Check sheet for the modelled part. Datum: model origin and axes. Units: mm. Round coordinates to 2 decimals unless told otherwise and drop trailing zeros. Write each loop counter-clockwise with the first axis right and the second up, starting at its lowest first coordinate (ties: lowest second). Pieces come first, ordered by that corner, then holes. Notation, with made-up numbers: (-17.75, -3.5) -> (21.25, -3.5) arc R23 cw to (21.25, 32.5) -> close; hole circle Ø1 at (58, 22). An arc over 180 degrees is marked (long way). Write item = value, one per line.
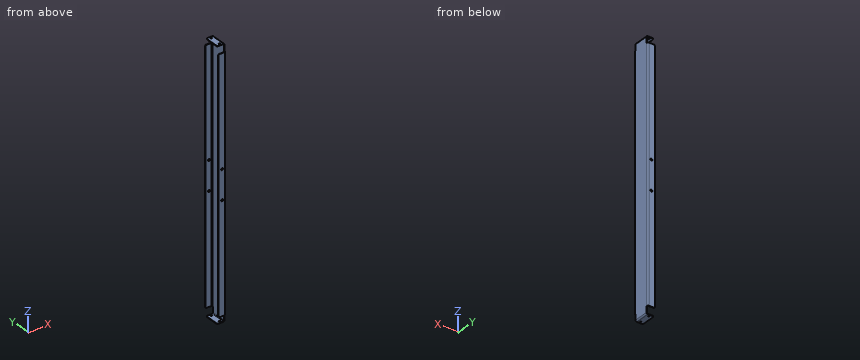
from build123d import *

# Parameters (mm, degrees)
SKETCH1_W                      = 861.06
SKETCH1_H                      = 63.5
BASE_FLANGE1_DEPTH             = 1.89738
EDGE_FLANGE1_STRIP_W           = 12.66952
EDGE_FLANGE1_STRIP_H           = 1.89738
EDGE_FLANGE1_STRIP_CUT_DEPTH   = 861.06
EDGE_FLANGE1_STRIP_2_W         = 12.66952
EDGE_FLANGE1_STRIP_2_H         = 1.89738
EDGE_FLANGE1_STRIP_CUT_2_DEPTH = 861.06
EDGE_FLANGE1_DEPTH             = 861.06
EDGE_FLANGE1_BEND_DEPTH        = 861.06
SKETCH12_W                     = 24.765
SKETCH12_H                     = 50.8
BOSS_EXTRUDE1_DEPTH            = 1.89738
SKETCH13_R                     = 3.3655
CUT_EXTRUDE1_DEPTH             = 461.403026733
EDGE_FLANGE2_STRIP_W           = 12.66952
EDGE_FLANGE2_STRIP_H           = 1.89738
EDGE_FLANGE2_STRIP_CUT_DEPTH   = 50.8
EDGE_FLANGE2_STRIP_2_W         = 12.66952
EDGE_FLANGE2_STRIP_2_H         = 1.89738
EDGE_FLANGE2_STRIP_CUT_2_DEPTH = 50.8
EDGE_FLANGE2_DEPTH             = 50.8
EDGE_FLANGE2_BEND_DEPTH        = 50.8
SKETCH20_R                     = 2.4638
CUT_EXTRUDE2_DEPTH             = 914.154728455
CHAMFER1_SIZE                  = 2.54


# Sheet-metal steps are written as plain solids
with BuildPart() as part:
    # Sketch1 → Base-Flange1 (new body)
    with BuildSketch(Plane(origin=(0, 0, 0), x_dir=(0, 0, -1), z_dir=(1, 0, 0))):
        with Locations((0, 31.75)):
            Rectangle(SKETCH1_W, SKETCH1_H)
    extrude(amount=-BASE_FLANGE1_DEPTH)

    # Edge-Flange1 strip (across the edge) → Edge-Flange1 strip cut (cut)
    with BuildSketch(Plane(origin=(-1.89738, 63.5, 430.53), x_dir=(0, -1, 0), z_dir=(0, 0, -1))):
        with Locations((-1.89738, -0.94869)):
            Rectangle(EDGE_FLANGE1_STRIP_W, EDGE_FLANGE1_STRIP_H)
    extrude(amount=EDGE_FLANGE1_STRIP_CUT_DEPTH, mode=Mode.SUBTRACT)

    # Edge-Flange1 strip 2 (across the edge) → Edge-Flange1 strip cut 2 (cut)
    with BuildSketch(Plane(origin=(-1.89738, 0, -430.53), x_dir=(0, 1, 0), z_dir=(0, 0, 1))):
        with Locations((-1.89738, -0.94869)):
            Rectangle(EDGE_FLANGE1_STRIP_2_W, EDGE_FLANGE1_STRIP_2_H)
    extrude(amount=EDGE_FLANGE1_STRIP_CUT_2_DEPTH, mode=Mode.SUBTRACT)

    # Edge-Flange1 section (across the edge) → Edge-Flange1 (add)
    with BuildSketch(Plane(origin=(-1.89738, 63.5, 430.53), x_dir=(0, -1, 0), z_dir=(0, 0, -1))):
        with BuildLine():
            Line((0, 2.54), (0, 23.50262))
            Line((0, 23.50262), (1.89738, 23.50262))
            Line((1.89738, 23.50262), (1.89738, 2.54))
            ThreePointArc((1.89738, 2.54), (2.641328776, 0.743948776), (4.43738, 0))
            Line((4.43738, 0), (4.43738, -1.89738))
            ThreePointArc((4.43738, -1.89738), (1.299678511, -0.597701489), (0, 2.54))
        make_face()
    extrude(amount=EDGE_FLANGE1_DEPTH)

    # Edge-Flange1 section 2 (across the edge) → Edge-Flange1 bend (add)
    with BuildSketch(Plane(origin=(-1.89738, 0, -430.53), x_dir=(0, 1, 0), z_dir=(0, 0, 1))):
        with BuildLine():
            Line((0, 2.54), (0, 23.50262))
            Line((0, 23.50262), (1.89738, 23.50262))
            Line((1.89738, 23.50262), (1.89738, 2.54))
            ThreePointArc((1.89738, 2.54), (2.641328776, 0.743948776), (4.43738, 0))
            Line((4.43738, 0), (4.43738, -1.89738))
            ThreePointArc((4.43738, -1.89738), (1.299678511, -0.597701489), (0, 2.54))
        make_face()
    extrude(amount=EDGE_FLANGE1_BEND_DEPTH)

    # Sketch12 → Boss-Extrude1 (add)
    with BuildSketch(Plane(origin=(0, 0, 0), x_dir=(0, 0, -1), z_dir=(1, 0, 0))):
        with Locations((-442.9125, 31.75)):
            Rectangle(SKETCH12_W, SKETCH12_H)
    boss_extrude1 = extrude(amount=-BOSS_EXTRUDE1_DEPTH)

    # Mirror1: Boss-Extrude1 across plane
    add(boss_extrude1.mirror(Plane.XY))

    # Sketch13 → Cut-Extrude1 (cut, through all)
    with BuildSketch(Plane(origin=(0, 63.5, 0), x_dir=(1, 0, 0), z_dir=(0, 1, 0))):
        with Locations(Location((-12.7, 50.8, 0), (0, 0, 180))):
            Circle(SKETCH13_R)
        with Locations(Location((-12.7, -50.8, 0), (0, 0, 180))):
            Circle(SKETCH13_R)
    extrude(amount=-CUT_EXTRUDE1_DEPTH, mode=Mode.SUBTRACT)

    # Edge-Flange2 strip (across the edge) → Edge-Flange2 strip cut (cut)
    with BuildSketch(Plane(origin=(-1.89738, 6.35, 455.295), x_dir=(0, 0, -1), z_dir=(0, 1, 0))):
        with Locations((-1.89738, -0.94869)):
            Rectangle(EDGE_FLANGE2_STRIP_W, EDGE_FLANGE2_STRIP_H)
    extrude(amount=EDGE_FLANGE2_STRIP_CUT_DEPTH, mode=Mode.SUBTRACT)

    # Edge-Flange2 strip 2 (across the edge) → Edge-Flange2 strip cut 2 (cut)
    with BuildSketch(Plane(origin=(-1.89738, 57.15, -455.295), x_dir=(0, 0, 1), z_dir=(0, -1, 0))):
        with Locations((-1.89738, -0.94869)):
            Rectangle(EDGE_FLANGE2_STRIP_2_W, EDGE_FLANGE2_STRIP_2_H)
    extrude(amount=EDGE_FLANGE2_STRIP_CUT_2_DEPTH, mode=Mode.SUBTRACT)

    # Edge-Flange2 section (across the edge) → Edge-Flange2 (add)
    with BuildSketch(Plane(origin=(-1.89738, 6.35, 455.295), x_dir=(0, 0, -1), z_dir=(0, 1, 0))):
        with BuildLine():
            Line((0, 2.54), (0, 23.50262))
            Line((0, 23.50262), (1.89738, 23.50262))
            Line((1.89738, 23.50262), (1.89738, 2.54))
            ThreePointArc((1.89738, 2.54), (2.641328776, 0.743948776), (4.43738, 0))
            Line((4.43738, 0), (4.43738, -1.89738))
            ThreePointArc((4.43738, -1.89738), (1.299678511, -0.597701489), (0, 2.54))
        make_face()
    extrude(amount=EDGE_FLANGE2_DEPTH)

    # Edge-Flange2 section 2 (across the edge) → Edge-Flange2 bend (add)
    with BuildSketch(Plane(origin=(-1.89738, 57.15, -455.295), x_dir=(0, 0, 1), z_dir=(0, -1, 0))):
        with BuildLine():
            Line((0, 2.54), (0, 23.50262))
            Line((0, 23.50262), (1.89738, 23.50262))
            Line((1.89738, 23.50262), (1.89738, 2.54))
            ThreePointArc((1.89738, 2.54), (2.641328776, 0.743948776), (4.43738, 0))
            Line((4.43738, 0), (4.43738, -1.89738))
            ThreePointArc((4.43738, -1.89738), (1.299678511, -0.597701489), (0, 2.54))
        make_face()
    extrude(amount=EDGE_FLANGE2_BEND_DEPTH)

    # Sketch20 → Cut-Extrude2 (cut, through all)
    with BuildSketch(Plane.XY.offset(455.295)):
        with Locations((-12.7, 50.8)):
            Circle(SKETCH20_R)
        with Locations((-12.7, 12.7)):
            Circle(SKETCH20_R)
    extrude(amount=-CUT_EXTRUDE2_DEPTH, mode=Mode.SUBTRACT)

    # Chamfer1
    chamfer1_edges = [part.edges().sort_by_distance(p)[0] for p in [
        (-25.4, 6.35, 454.34631),
        (-25.4, 57.15, 454.34631),
        (-25.4, 57.15, -454.34631),
        (-25.4, 6.35, -454.34631),
        (-25.4, 62.55131, 430.53),
        (-25.4, 62.55131, -430.53),
        (-25.4, 0.94869, -430.53),
        (-25.4, 0.94869, 430.53),
    ]]
    chamfer(chamfer1_edges, length=CHAMFER1_SIZE)


solid = part.part
(1) Material ranges on L1, parallel to Y at x = -12.7, z = 454.7; L2, parallel to Z at x = -12.7, y = 0.95; L3, parallel to Y at x = -7.5, z = -47, recorded low to high. Write a range as [from, to].
Worked answers:
L1 = [6.35, 10.24], [15.16, 48.34], [53.26, 57.15]
L2 = [-430.53, -54.17], [-47.43, 47.43], [54.17, 430.53]
L3 = [0, 1.9], [61.6, 63.5]
(2) Sectioned sample at B-B on y = 32. Enter the section's corners in (x, z) (3 decimals), then the cut area to 3 significant figures.
Worked answers:
outline = (-25.4, -455.295) -> (-4.437, -455.295) arc R4.437 ccw to (0, -450.858) -> (0, 450.858) arc R4.437 ccw to (-4.437, 455.295) -> (-25.4, 455.295) -> (-25.4, 453.398) -> (-4.437, 453.398) arc R2.54 cw to (-1.897, 450.858) -> (-1.897, -450.858) arc R2.54 cw to (-4.437, -453.398) -> (-25.4, -453.398) -> close
area = 1,810 mm²
(3) Go/stop test with flat-tipped pins: P1, Ø4.5, axis at x = -12.7, y = 50.8, coming from the +Z side; P2, Ø3, axis at y = 33.5, z = 101, coming from the -X side. Record where each tip stops, or that it passes through.
Worked answers:
P1 = through
P2 = -1.9
(4) Sectioned sample at A-A on z = -79. Enter the section's corners in (x, y), then the cut area to 3 significant figures.
Worked answers:
outline = (-25.4, 0) -> (-4.44, 0) arc R4.44 ccw to (0, 4.44) -> (0, 59.06) arc R4.44 ccw to (-4.44, 63.5) -> (-25.4, 63.5) -> (-25.4, 61.6) -> (-4.44, 61.6) arc R2.54 cw to (-1.9, 59.06) -> (-1.9, 4.44) arc R2.54 cw to (-4.44, 1.9) -> (-25.4, 1.9) -> close
area = 204 mm²
